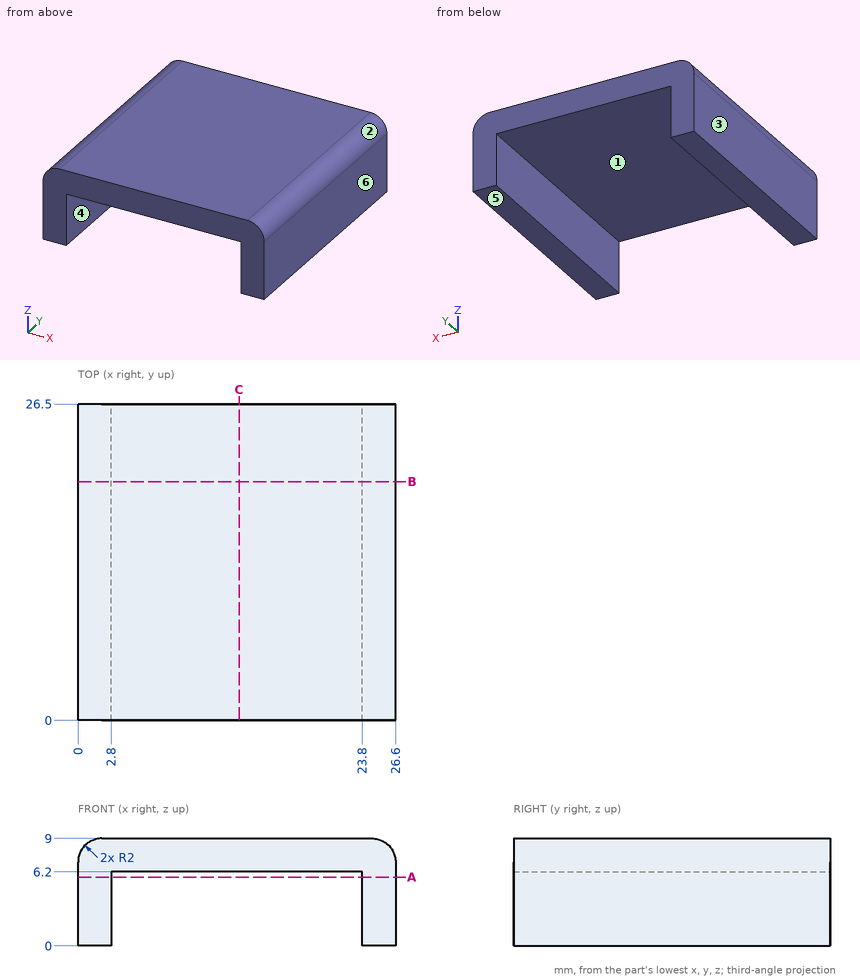
Here's the drawing with two shaded views (mm, measured from the low corner). I have some questions. A direction names the side the tool comes from. Coordinates: 2 decimals unless noted, no trailing zeros. Write each loop counter-clockwise with the first axis right and the second up, starting at its lowest first coordinate (ties: lowest second). Pieces come first, ordered by that corner, then holes. Notation, with made-up numbers: (1.25, 73.25) -> (36.25, 73.25) arc R22 cw to (36.25, 106.25) -> close; hole circle Ø3 at (76.5, 35.5). An arc over 180 degrees is marked (long way). Use a Markdown table: item, result. Add a question column.
(1) We'd pull the mould along X, two halves only. Please class the marked faces 3, 4, 5 and 6: +X half, -X half, draft (parallel to the pull), parting line (faces both ways), or undercut.
(2) For the marked faces 1 and 2, which set-ups out of +Z, -Z, +X, -X, +Y, -Y let a thin tool reach every point of the face, with its end or its side?
(3) I'm going to push a flat-ended pin straight in: P1, Ø6.5, axis at x = 17, y = 11.5, coming from the -Z side. Where does the tip first touch, or does it pass through?
(4) Please list where these lines run through material, in increasing order: line 1 (X direction, y = 13, z = 3.5); line 2 (Z direction, x = 13.75, y = 7.5); line 3 (Z direction, x = 25.25, y = 12.25).
(5) If we section it at A-A, the plane z = 5.75: Write out the boundary of the cut face in (x, y).
(6) If we section it at C-C, the plane x = 13.5: Write out the boundary of the cut face in (y, z).
(7) If we section it at B-B, the plane y = 20: Write out the boundary of the cut face in (x, z).
Outcome:
| question | item | result |
|---|---|---|
| 1 | face 3 | -X half |
| 1 | face 4 | undercut |
| 1 | face 5 | draft |
| 1 | face 6 | +X half |
| 2 | face 1 | -Z, +Y, -Y |
| 2 | face 2 | +Z, +X, +Y, -Y |
| 3 | P1 | stops at z = 6.2 |
| 4 | line 1 | x = 0 to 2.8, 23.8 to 26.6 |
| 4 | line 2 | z = 6.2 to 9 |
| 4 | line 3 | z = 0 to 8.89 |
| 5 | outline | (0, 0) -> (2.8, 0) -> (2.8, 26.5) -> (0, 26.5) -> close; (23.8, 0) -> (26.6, 0) -> (26.6, 26.5) -> (23.8, 26.5) -> close |
| 6 | outline | (0, 6.2) -> (26.5, 6.2) -> (26.5, 9) -> (0, 9) -> close |
| 7 | outline | (0, 0) -> (2.8, 0) -> (2.8, 6.2) -> (23.8, 6.2) -> (23.8, 0) -> (26.6, 0) -> (26.6, 7) arc R2 ccw to (24.6, 9) -> (2, 9) arc R2 ccw to (0, 7) -> close |
